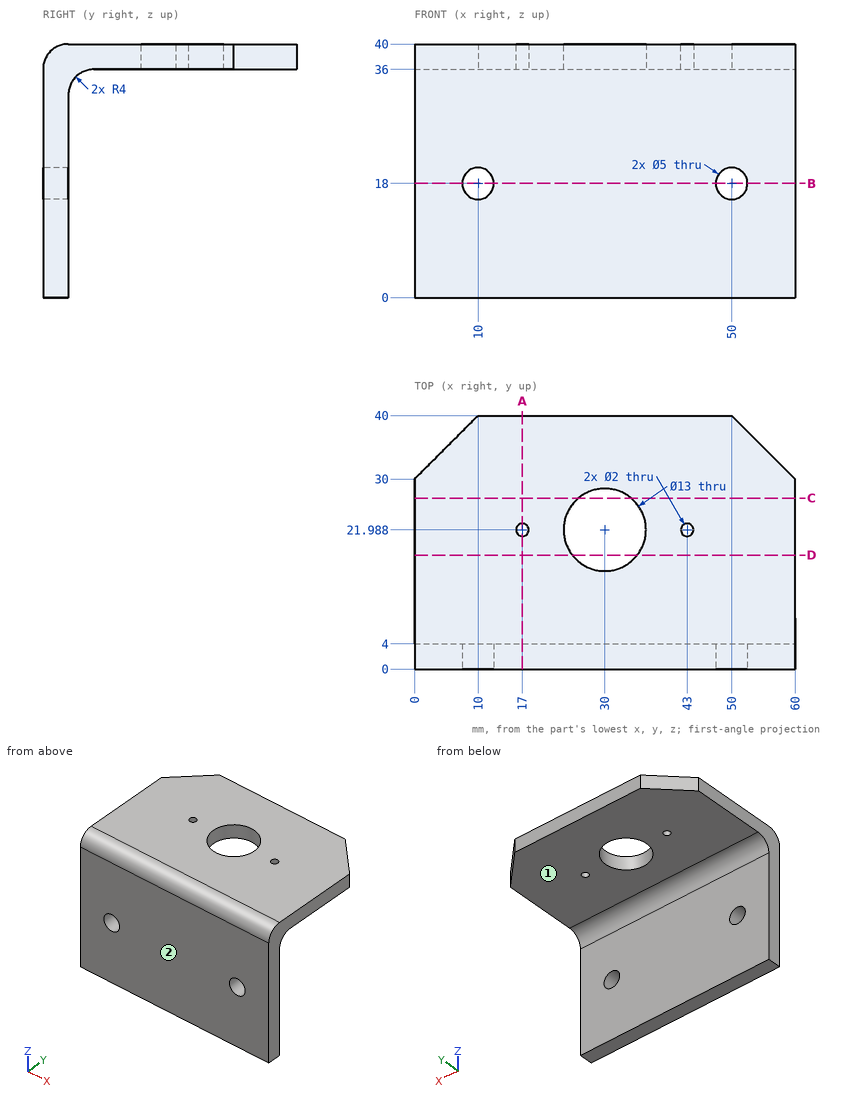
Geometry check sheet. Reference: drawing and pictorial views, mm from the part's lowest x, y, z. A direction names the side the tool comes from. Give positions to 0.01 mm unless a question says otherwise; leave off trailing zeros. Loops run counter-clockwise (first coordinate to the right, second up) from the corner with the lowest first, then second, coordinate; pieces in that order, holes last.
1. Section check C-C, the plane y = 27. Enter the section's corners in (x, z), then the cut area to 3 significant figures.
2. Thickness scan on line 1 (X direction, y = 1, z = 18); line 2 (Y direction, x = 28, z = 15); line 3 (Z direction, x = 41, y = 14). Record the ranges inside material, lowest first.
3. Section check A-A, the plane x = 17. Enter the section's corners in (y, z).
4. Section check B-B, the plane z = 18. Enter the section's corners in (x, y).
5. Set-up check for the marked faces 1 and 2: record each of +Z, -Z, +X, -X, +Y, -Y from which the full face is reachable in a straight line by a thin tool's end or side.
6. Go/stop test with flat-tipped pins: pin 1 Ø1 at (x, z) = (22, 8.5) entering from +Y; pin 2 Ø3 at (x, y) = (43, 21.99) entering from -Z; pin 3 Ø1 at (x, z) = (23.5, 33) entering from +Y. Record where each tip stops, or that it passes through.
7. Section check D-D, the plane y = 18. Enter the section's corners in (x, z).
Geometry says:
1. outline: (0, 36) - (25.86, 36) - (25.86, 40) - (0, 40) - close; (34.14, 36) - (60, 36) - (60, 40) - (34.14, 40) - close
1. area: 207 mm2
2. line 1: x = 0 to 7.5, 12.5 to 47.5, 52.5 to 60
2. line 2: y = 0 to 4
2. line 3: z = 36 to 40
3. outline: (0, 0) - (4, 0) - (4, 32) arc R4 cw to (8, 36) - (20.99, 36) - (20.99, 40) - (4, 40) arc R4 ccw to (0, 36) - close; (22.99, 36) - (40, 36) - (40, 40) - (22.99, 40) - close
4. outline: (0, 0) - (7.5, 0) - (7.5, 4) - (0, 4) - close; (12.5, 0) - (47.5, 0) - (47.5, 4) - (12.5, 4) - close; (52.5, 0) - (60, 0) - (60, 4) - (52.5, 4) - close
5. face 1: -Z, +X, -X, +Y
5. face 2: +Z, -Z, +X, -X, -Y
6. pin 1: stops at y = 4
6. pin 2: stops at z = 36
6. pin 3: stops at y = 4.29
7. outline: (0, 36) - (24.87, 36) - (24.87, 40) - (0, 40) - close; (35.13, 36) - (60, 36) - (60, 40) - (35.13, 40) - close
